```python
from build123d import *

# Parameters (mm, degrees)
ESQUISSE1_W                  = 478
ESQUISSE1_H                  = 68.5
BOSS_EXTRU_1_DEPTH           = 15
ENL_V_MAT_EXTRU_1_DEPTH      = 484.116186854
ENL_V_MAT_EXTRU_1_DEPTH_BACK = 484.116186854
ESQUISSE2_R                  = 4.25
ENL_V_MAT_EXTRU_2_DEPTH      = 484.116186854
ENL_V_MAT_EXTRU_2_DEPTH_BACK = 484.116186854
ESQUISSE3_R                  = 19.5
ENL_V_MAT_EXTRU_3_DEPTH      = 484.116186854
ENL_V_MAT_EXTRU_3_DEPTH_BACK = 484.116186854
ESQUISSE4_W                  = 30
ESQUISSE4_H                  = 8.75


with BuildPart() as part:
    # Esquisse1 → Boss.-Extru.1 (new body)
    with BuildSketch(Plane.XY):
        with Locations((239, 34.25)):
            Rectangle(ESQUISSE1_W, ESQUISSE1_H)
    extrude(amount=BOSS_EXTRU_1_DEPTH)

    # Esquisse2 → Enlèv. mat.-Extru.1 (cut, two sides: drawn at the far end of the back side and taken through both)
    with BuildSketch(Plane.XY.offset(15).offset(-ENL_V_MAT_EXTRU_1_DEPTH_BACK)):
        with Locations((227.5, 58.25)):
            Circle(ESQUISSE2_R)
        with Locations(Location((227.5, 10.25, 0), (0, 0, 180))):
            Circle(ESQUISSE2_R)
        with Locations((179.5, 10.25)):
            Circle(ESQUISSE2_R)
        with Locations(Location((179.5, 58.25, 0), (0, 0, 180))):
            Circle(ESQUISSE2_R)
        with Locations((156.5, 58.25)):
            Circle(ESQUISSE2_R)
        with Locations(Location((156.5, 10.25, 0), (0, 0, 180))):
            Circle(ESQUISSE2_R)
        with Locations((108.5, 10.25)):
            Circle(ESQUISSE2_R)
        with Locations(Location((108.5, 58.25, 0), (0, 0, 180))):
            Circle(ESQUISSE2_R)
        with Locations((85.5, 58.25)):
            Circle(ESQUISSE2_R)
        with Locations(Location((85.5, 10.25, 0), (0, 0, 180))):
            Circle(ESQUISSE2_R)
        with Locations((37.5, 10.25)):
            Circle(ESQUISSE2_R)
        with Locations(Location((37.5, 58.25, 0), (0, 0, 180))):
            Circle(ESQUISSE2_R)
        with Locations((440.5, 58.25)):
            Circle(ESQUISSE2_R)
        with Locations(Location((440.5, 10.25, 0), (0, 0, 180))):
            Circle(ESQUISSE2_R)
        with Locations((392.5, 10.25)):
            Circle(ESQUISSE2_R)
        with Locations(Location((392.5, 58.25, 0), (0, 0, 180))):
            Circle(ESQUISSE2_R)
        with Locations((369.5, 58.25)):
            Circle(ESQUISSE2_R)
        with Locations(Location((369.5, 10.25, 0), (0, 0, 180))):
            Circle(ESQUISSE2_R)
        with Locations((321.5, 10.25)):
            Circle(ESQUISSE2_R)
        with Locations(Location((321.5, 58.25, 0), (0, 0, 180))):
            Circle(ESQUISSE2_R)
        with Locations((298.5, 58.25)):
            Circle(ESQUISSE2_R)
        with Locations(Location((298.5, 10.25, 0), (0, 0, 180))):
            Circle(ESQUISSE2_R)
        with Locations((250.5, 10.25)):
            Circle(ESQUISSE2_R)
        with Locations(Location((250.5, 58.25, 0), (0, 0, 180))):
            Circle(ESQUISSE2_R)
    extrude(amount=ENL_V_MAT_EXTRU_1_DEPTH + ENL_V_MAT_EXTRU_1_DEPTH_BACK, mode=Mode.SUBTRACT)

    # Esquisse3 → Enlèv. mat.-Extru.2 (cut, two sides: drawn at the far end of the back side and taken through both)
    with BuildSketch(Plane.XY.offset(15).offset(-ENL_V_MAT_EXTRU_2_DEPTH_BACK)):
        with Locations((203.5, 34.25)):
            Circle(ESQUISSE3_R)
        with Locations((132.5, 34.25)):
            Circle(ESQUISSE3_R)
        with Locations((61.5, 34.25)):
            Circle(ESQUISSE3_R)
        with Locations(Location((416.5, 34.25, 0), (0, 0, 180))):
            Circle(ESQUISSE3_R)
        with Locations(Location((345.5, 34.25, 0), (0, 0, 180))):
            Circle(ESQUISSE3_R)
        with Locations(Location((274.5, 34.25, 0), (0, 0, 180))):
            Circle(ESQUISSE3_R)
    extrude(amount=ENL_V_MAT_EXTRU_2_DEPTH + ENL_V_MAT_EXTRU_2_DEPTH_BACK, mode=Mode.SUBTRACT)

    # Esquisse4 → Enlèv. mat.-Extru.3 (cut, two sides: drawn at the far end of the back side and taken through both)
    with BuildSketch(Plane.XY.offset(15).offset(-ENL_V_MAT_EXTRU_3_DEPTH_BACK)):
        with Locations((15, 4.375)):
            Rectangle(ESQUISSE4_W, ESQUISSE4_H)
        with Locations((463, 4.375)):
            Rectangle(ESQUISSE4_W, ESQUISSE4_H)
    extrude(amount=ENL_V_MAT_EXTRU_3_DEPTH + ENL_V_MAT_EXTRU_3_DEPTH_BACK, mode=Mode.SUBTRACT)


solid = part.part
```
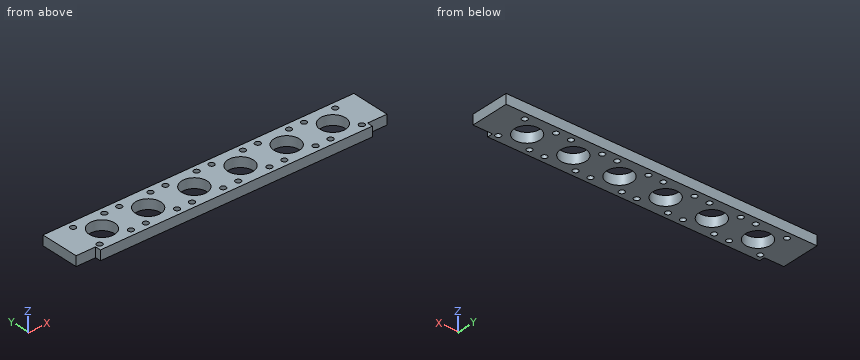
Input: part model. Units: mm. Frame: model coordinates. Give positions to 0.01 mm unless a question says otherwise; leave off trailing zeros. Order: outer loops, then holes, each group sorted by start corner. A loop starts at its lowest first (then second) coordinate and runs counter-clockwise, first axis right, second up.
1. Cut plane A-A (x = 345.5). Return loops of the section in (y, z).
Computed:
outline: (0, 0) - (14.75, 0) - (14.75, 15) - (0, 15) - close; (53.75, 0) - (68.5, 0) - (68.5, 15) - (53.75, 15) - close
2. Cut plane D-D (z = 4.25). State how many separate pieces and enclosed holes the cut face has, and give its area (3 significant figures).
Computed:
separate pieces: 1
enclosed holes: 30
area: 23,700 mm2
3. Line query: probe 1 along Y at (x, z) = (37.5, 10.5); probe 2 along Y at (x, z) = (274.5, 4.5); probe 3 along Y at (x, z) = (438, 6.5). Output: solid intervals per line, ascending.
Computed:
probe 1: y = 0 to 6, 14.5 to 54, 62.5 to 68.5
probe 2: y = 0 to 14.75, 53.75 to 68.5
probe 3: y = 0 to 6.81, 13.69 to 54.81, 61.69 to 68.5
4. Cut plane B-B (x = 108.5). Return loops of the section in (y, z).
Computed:
outline: (0, 0) - (6, 0) - (6, 15) - (0, 15) - close; (14.5, 0) - (54, 0) - (54, 15) - (14.5, 15) - close; (62.5, 0) - (68.5, 0) - (68.5, 15) - (62.5, 15) - close
5. Pin query (flat end, axial travel): pin 1 Ø2.5 at (y, z) = (2.5, 5.5) entering from -X. Return the tip coordinate at first contact, or that it passes through.
Computed:
pin 1: stops at x = 30
6. Cut plane C-C (y = 25.5). Return loops of the section in (x, z).
Computed:
outline: (0, 0) - (44.07, 0) - (44.07, 15) - (0, 15) - close; (78.93, 0) - (115.07, 0) - (115.07, 15) - (78.93, 15) - close; (149.93, 0) - (186.07, 0) - (186.07, 15) - (149.93, 15) - close; (220.93, 0) - (257.07, 0) - (257.07, 15) - (220.93, 15) - close; (291.93, 0) - (328.07, 0) - (328.07, 15) - (291.93, 15) - close; (362.93, 0) - (399.07, 0) - (399.07, 15) - (362.93, 15) - close; (433.93, 0) - (478, 0) - (478, 15) - (433.93, 15) - close
